Source: CAD feature listing. Evaluate the final solid. Frame: model axes, mm. Face numbers are marked on the shaded views. A direction names the side the tool comes from. Round coordinates to 2 decimals unless told otherwise and drop trailing zeros. Loops run counter-clockwise (first coordinate to the right, second up) from the corner with the lowest first, then second, coordinate; pieces in that order, holes last. Notation, with made-up numbers: M 26.5,6 L 82.5,6 A16 cw 82.5,26 Z; hole C -24,9.25 d11. An arc over 180 degrees is marked long. One line per item, written item: value.
from build123d import *

# Parameters (mm, degrees)
BOSS_EXTRUDE1_DEPTH      = 22
BOSS_EXTRUDE1_DEPTH_BACK = 22
SKETCH2_W                = 38
SKETCH2_H                = 20
CUT_EXTRUDE1_DEPTH       = 105.423416914
SKETCH3_W                = 7
SKETCH3_H                = 44
BOSS_EXTRUDE2_DEPTH      = 65.5
SKETCH23_R               = 5
SKETCH23_R_2             = 1.2
CUT_EXTRUDE2_DEPTH       = 111.605436123
SKETCH24_W               = 28.5
SKETCH24_H               = 34
CUT_EXTRUDE3_DEPTH       = 90.954502389
SKETCH26_R               = 1.2
SKETCH26_R_2             = 5
SKETCH26_R_3             = 1.45
CUT_EXTRUDE6_DEPTH       = 107.330263801
SKETCH27_W               = 29.7
SKETCH27_H               = 35.2
CUT_EXTRUDE8_DEPTH       = 73.137455597
SKETCH29_W               = 7
SKETCH29_H               = 35
CUT_EXTRUDE10_DEPTH      = 74.468530678
CHAMFER2_SIZE            = 5
FILLET1_START            = -23
FILLET1_DEPTH            = 46


with BuildPart() as part:
    # Sketch1 → Boss-Extrude1 (new, two sides: drawn at the far end of the back side and taken through both)
    with BuildSketch(Plane.XY.offset(-BOSS_EXTRUDE1_DEPTH_BACK)):
        with BuildLine():
            Line((10.25, -60), (10.25, 0))
            ThreePointArc((10.25, 0), (0, -10.25), (-10.25, 0))
            Line((-10.25, 0), (-10.25, -60))
            Line((-10.25, -60), (-10.25, -100))
            Line((-10.25, -100), (10.25, -100))
            Line((10.25, -100), (10.25, -60))
        make_face()
        with BuildLine():
            Line((10.25, 0), (9.2, 0))
            ThreePointArc((9.2, 0), (8.816088231, -0.879772698), (7.91, -1.196620241))
            ThreePointArc((7.91, -1.196620241), (5.656854249, -5.656854249), (1.196620241, -7.91))
            ThreePointArc((1.196620241, -7.91), (1.199154762, -7.954968281), (1.2, -8))
            ThreePointArc((1.2, -8), (-0.045031719, -9.199154762), (-1.196620241, -7.91))
            ThreePointArc((-1.196620241, -7.91), (-5.656854249, -5.656854249), (-7.91, -1.196620241))
            ThreePointArc((-7.91, -1.196620241), (-8.816088231, -0.879772698), (-9.2, 0))
            Line((-9.2, 0), (-10.25, 0))
            ThreePointArc((-10.25, 0), (0, -10.25), (10.25, 0))
        make_face()
        with BuildLine():
            ThreePointArc((7.91, -1.196620241), (7.120227302, -0.816088231), (6.8, 0))
            Line((6.8, 0), (4.2, 0))
            ThreePointArc((4.2, 0), (0, -4.2), (-4.2, 0))
            Line((-4.2, 0), (-6.8, 0))
            ThreePointArc((-6.8, 0), (-7.120227302, -0.816088231), (-7.91, -1.196620241))
            ThreePointArc((-7.91, -1.196620241), (-5.656854249, -5.656854249), (-1.196620241, -7.91))
            ThreePointArc((-1.196620241, -7.91), (0, -6.8), (1.196620241, -7.91))
            ThreePointArc((1.196620241, -7.91), (5.656854249, -5.656854249), (7.91, -1.196620241))
        make_face()
        with BuildLine():
            Line((4.2, 0), (6.8, 0))
            ThreePointArc((6.8, 0), (7.120227302, 0.816088231), (7.91, 1.196620241))
            ThreePointArc((7.91, 1.196620241), (5.656854249, 5.656854249), (1.196620241, 7.91))
            ThreePointArc((1.196620241, 7.91), (0, 6.8), (-1.196620241, 7.91))
            ThreePointArc((-1.196620241, 7.91), (-5.656854249, 5.656854249), (-7.91, 1.196620241))
            ThreePointArc((-7.91, 1.196620241), (-7.120227302, 0.816088231), (-6.8, 0))
            Line((-6.8, 0), (-4.2, 0))
            ThreePointArc((-4.2, 0), (0, 4.2), (4.2, 0))
        make_face()
        with BuildLine():
            ThreePointArc((7.91, 1.196620241), (8.816088231, 0.879772698), (9.2, 0))
            Line((9.2, 0), (10.25, 0))
            ThreePointArc((10.25, 0), (0, 10.25), (-10.25, 0))
            Line((-10.25, 0), (-9.2, 0))
            ThreePointArc((-9.2, 0), (-8.816088231, 0.879772698), (-7.91, 1.196620241))
            ThreePointArc((-7.91, 1.196620241), (-5.656854249, 5.656854249), (-1.196620241, 7.91))
            ThreePointArc((-1.196620241, 7.91), (-0.045031719, 9.199154762), (1.2, 8))
            ThreePointArc((1.2, 8), (1.199154762, 7.954968281), (1.196620241, 7.91))
            ThreePointArc((1.196620241, 7.91), (5.656854249, 5.656854249), (7.91, 1.196620241))
        make_face()
    extrude(amount=BOSS_EXTRUDE1_DEPTH + BOSS_EXTRUDE1_DEPTH_BACK)

    # Sketch2 → Cut-Extrude1 (cut, through all)
    with BuildSketch(Plane.ZY.offset(10.25)):
        with Locations((0, 0.25)):
            Rectangle(SKETCH2_W, SKETCH2_H)
    extrude(amount=-CUT_EXTRUDE1_DEPTH, mode=Mode.SUBTRACT)

    # Sketch3 → Boss-Extrude2 (add)
    with BuildSketch(Plane(origin=(0, -9.75, 0), x_dir=(1, 0, 0), z_dir=(0, 1, 0))):
        with Locations((-13.75, 0)):
            Rectangle(SKETCH3_W, SKETCH3_H)
        with Locations((13.75, 0)):
            Rectangle(SKETCH3_W, SKETCH3_H)
    extrude(amount=-BOSS_EXTRUDE2_DEPTH)

    # Sketch23 → Cut-Extrude2 (cut, through all)
    with BuildSketch(Plane.XY.offset(22)):
        with BuildLine():
            Line((-10.25, -100), (10.25, -100))
            Line((10.25, -100), (10.25, -85))
            ThreePointArc((10.25, -85), (0, -95.25), (-10.25, -85))
            Line((-10.25, -85), (-10.25, -100))
        make_face()
        with Locations((0, -85)):
            Circle(SKETCH23_R)
        with Locations((8, -85)):
            Circle(SKETCH23_R_2)
        with Locations((0, -77)):
            Circle(SKETCH23_R_2)
        with Locations((0, -93)):
            Circle(SKETCH23_R_2)
        with Locations((-8, -85)):
            Circle(SKETCH23_R_2)
    extrude(amount=-CUT_EXTRUDE2_DEPTH, mode=Mode.SUBTRACT)

    # Sketch24 → Cut-Extrude3 (cut, through all)
    with BuildSketch(Plane(origin=(0, -9.75, 0), x_dir=(1, 0, 0), z_dir=(0, 1, 0))):
        Rectangle(SKETCH24_W, SKETCH24_H)
    extrude(amount=-CUT_EXTRUDE3_DEPTH, mode=Mode.SUBTRACT)

    # Sketch26 → Cut-Extrude6 (cut, through all)
    # profile 1 of 5: a face of its own
    with BuildSketch(Plane.XY.offset(22)):
        with BuildLine():
            Line((10.25, -75.25), (14.25, -75.25))
            Line((14.25, -75.25), (14.25, -56.53282359))
            Line((14.25, -56.53282359), (14.25, -56.25))
            Line((14.25, -56.25), (-14.25, -56.25))
            Line((-14.25, -56.25), (-14.25, -56.53282359))
            Line((-14.25, -56.53282359), (-14.25, -75.25))
            Line((-14.25, -75.25), (-10.25, -75.25))
            Line((-10.25, -75.25), (-10.25, -85))
            ThreePointArc((-10.25, -85), (0, -95.25), (10.25, -85))
            Line((10.25, -85), (10.25, -75.25))
        make_face()
        with Locations((-8, -85)):
            Circle(SKETCH26_R, mode=Mode.SUBTRACT)
        with Locations((0, -85)):
            Circle(SKETCH26_R_2, mode=Mode.SUBTRACT)
        with Locations((0, -77)):
            Circle(SKETCH26_R, mode=Mode.SUBTRACT)
        with Locations((0, -93)):
            Circle(SKETCH26_R, mode=Mode.SUBTRACT)
        with Locations((8, -85)):
            Circle(SKETCH26_R, mode=Mode.SUBTRACT)
    # profile 2 of 5: a face of its own
    with BuildSketch(Plane.XY.offset(22)):
        Polygon((-17.25, -75.25), (-14.25, -75.25), (-14.25, -56.53282359), (-14.25, -56.25), (-17.25, -56.25), align=None)
    # profile 3 of 5: a face of its own
    with BuildSketch(Plane.XY.offset(22)):
        Polygon((14.25, -56.53282359), (14.25, -75.25), (17.25, -75.25), (17.25, -56.25), (14.25, -56.25), align=None)
    # profile 4 of 5: a face of its own
    with BuildSketch(Plane.XY.offset(22)):
        with Locations((-11, -53)):
            Circle(SKETCH26_R_3)
    # profile 5 of 5: a face of its own
    with BuildSketch(Plane.XY.offset(22)):
        with Locations((11, -53)):
            Circle(SKETCH26_R_3)
    extrude(amount=-CUT_EXTRUDE6_DEPTH, mode=Mode.SUBTRACT)

    # Sketch27 → Cut-Extrude8 (cut, through all)
    with BuildSketch(Plane.XZ.offset(56.25)):
        Rectangle(SKETCH27_W, SKETCH27_H)
    extrude(amount=-CUT_EXTRUDE8_DEPTH, mode=Mode.SUBTRACT)

    # Sketch29 → Cut-Extrude10 (cut, through all)
    with BuildSketch(Plane(origin=(0, 0, -22), x_dir=(-1, 0, 0), z_dir=(0, 0, -1))):
        with Locations((-13.75, -27.25)):
            Rectangle(SKETCH29_W, SKETCH29_H)
    extrude(amount=-CUT_EXTRUDE10_DEPTH, mode=Mode.SUBTRACT)

    # Chamfer2
    # the kernel refuses this chamfer: 5 mm, written as the material it takes off along each edge
    with BuildSketch(Plane(origin=(-17.25, -56.25, 34.85841494), x_dir=(1, 0, 0), z_dir=(0, 0, -1))) as chamfer2_piece_1:
        Polygon((CHAMFER2_SIZE, 0), (0, -CHAMFER2_SIZE), (0, 0), align=None)
    extrude(amount=69.71682988, mode=Mode.SUBTRACT)

    # Fillet1: read off the stored shape, not the designer's step
    # Fillet1 outline → Fillet1 (cut)
    with BuildSketch(Plane.XY.offset(FILLET1_START)):
        with BuildLine():
            ThreePointArc((10.25, -44.75), (15.312257748, -48.373312231), (17.25, -54.289392014))
            Line((17.25, -54.289392014), (17.25, -44.75))
            Line((17.25, -44.75), (10.25, -44.75))
        make_face()
    extrude(amount=FILLET1_DEPTH, mode=Mode.SUBTRACT)


solid = part.part
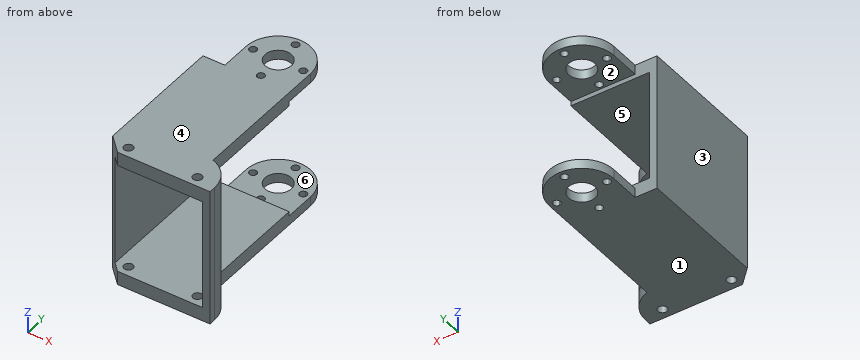
1. Reachability of the marked faces 4, 5 and 6 from +Z, -Z, +X, -X, +Y, -Y: full face, straight path, thin tool, end or side. Return the list, or none.
Report:
face 4: +Z, +X, -X, +Y, -Y
face 5: +Y, -Y
face 6: +X, -X, +Y
2. Section query A-A (x = -11). Return the cut outline in (y, z), and give its area (3 significant figures).
Report:
outline: M -56.25,-22 L -54.45,-22 L -54.45,-17.6 L -56.25,-17.6 Z; M -56.25,17.6 L -54.45,17.6 L -54.45,22 L -56.25,22 Z; M -51.55,-22 L -9.75,-22 L -9.75,-17.6 L -51.55,-17.6 Z; M -51.55,17.6 L -9.75,17.6 L -9.75,22 L -51.55,22 Z
area: 384 mm2
3. Ray query, line 1 (Z direction, x = -8, y = -8); line 2 (Z direction, x = -9, y = -22); line 3 (Y direction, x = 1, z = -20). Return the intervals inside material, ascending. Write a range as [from, to].
Report:
line 1: z = [-22, -19], [19, 22]
line 2: z = [-22, -17.6], [17.6, 22]
line 3: y = [-56.25, -8.66], [-7.34, -4.08], [4.08, 7.34], [8.66, 10.2]
4. Section query B-B (y = -34). Return the cut outline in (x, z).
Report:
outline: M -17.25,-22 L 10.25,-22 L 10.25,-17.6 L -14.85,-17.6 L -14.85,17.6 L 10.25,17.6 L 10.25,22 L -17.25,22 Z
5. Section query C-C (z = 5). Return the cut outline in (x, y).
Report:
outline: M -17.25,-51.25 L -14.85,-53.65 L -14.85,-9.75 L -17.25,-9.75 Z; M 14.85,-56.25 L 17.25,-56.25 L 17.25,-54.29 A10 ccw 14.85,-47.79 Z
6. Pull-direction query (Z, two-part tool) for the marked faces 1, 2 and 3; classes: released by +Z, released by -Z, zero draft, split by the parting line, or undercut.
Report:
face 1: released by -Z
face 2: undercut
face 3: zero draft
7. Pin query (flat end, axial travel): pin 1 (3.5 mm diameter, centred on y = -3, z = -20, fed in from -X); pin 2 (6 mm diameter, centred on x = -4, y = 0, fed in from -Z); pin 3 (2 mm diameter, centred on y = -23, z = -20, fed in from +X); pin 4 (17.5 mm diameter, centred on y = -36.5, z = 7.5, fed in from +X). Return the tip coordinate at first contact, or that it passes through.
Report:
pin 1: stops at x = -10.25
pin 2: stops at z = -22
pin 3: stops at x = 10.25
pin 4: stops at x = -14.85
8. Section query D-D (x = 14). Return the cut outline in (y, z).
Report:
outline: M -56.25,-22 L -46.91,-22 L -46.91,-17.6 L -56.25,-17.6 Z; M -56.25,17.6 L -46.91,17.6 L -46.91,22 L -56.25,22 Z
